The figure shows three views and two pictorial views of one solid part (mm, origin at its lowest corner). Answer the questions. A direction names the side the tool comes from. Round coordinates to 2 decimals unless told otherwise and drop trailing zeros. Answer as a JSON object with one key per item and string values. Group by question number.
Item 1: The mould has two halves that part along X. Classify the marked faces 4, 5 and 6: pulls with the +X half, pulls with the -X half, needs draft (parallel to the pull), parting line crosses it, or undercut.
Item 2: Section A-A, the plane z = 10 is taken. Count the separate pieces of the cut face and the enclosed holes in it, plus the area to 3 significant figures.
Item 3: Given P1, Ø11, axis at x = 7, y = 25.5, coming from the -Z side; P2, Ø6, axis at y = 24.5, z = 3.5, coming from the -X side; P3, Ø6, axis at x = 9.5, z = 6, coming from the -Y side, each flat-ended and moving along its own axis, determine where each tip first touches the part or whether it passes through.
Item 4: Consider probe 1 along Y at (x, z) = (28, 12.75); probe 2 along Z at (x, y) = (10, 13.5); probe 3 along Y at (x, z) = (5, 13.7). Determine where each line is inside the solid, lowest interval first. Write a range as from..to.
Item 5: For the marked faces 1, 2 and 3, determine the directions among +Z, -Z, +X, -X, +Y, -Y from which every point of the face is accessible in a straight line to the end or side of a thin tool.
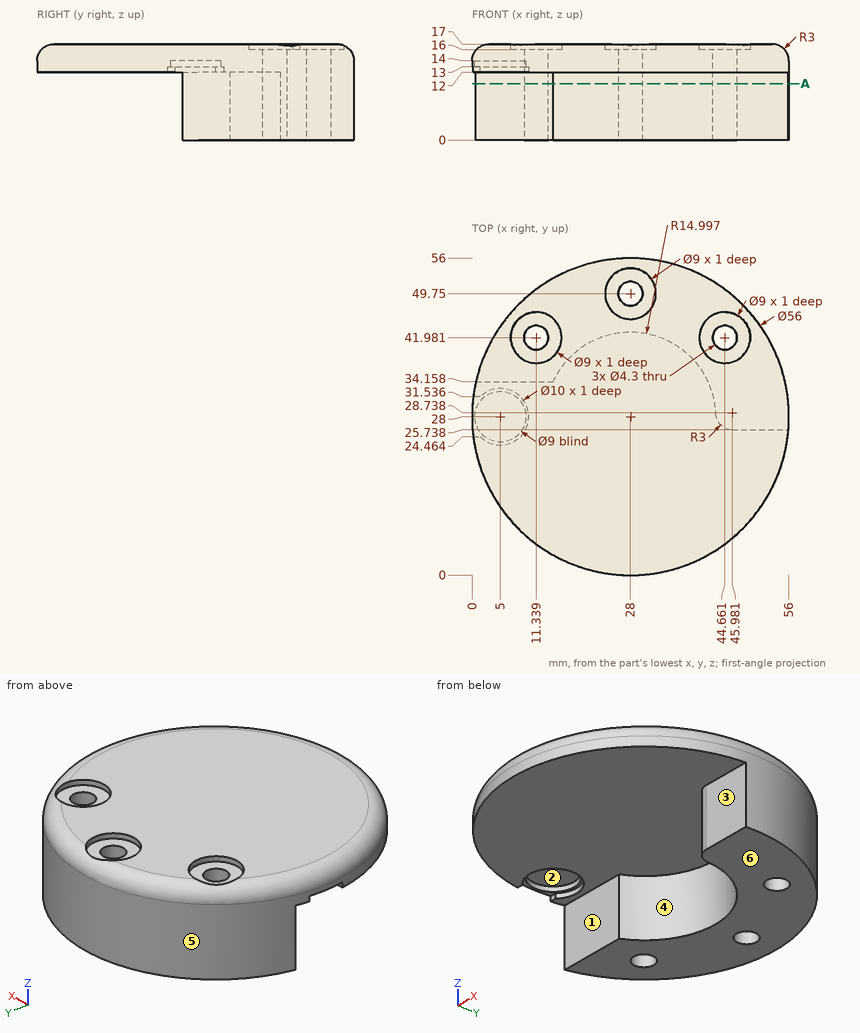
Values found:
{
 "1": {"face 4": "undercut", "face 5": "parting line crosses it", "face 6": "needs draft"},
 "2": {"separate pieces": "1", "enclosed holes": "3", "area": "781 mm2"},
 "3": {"P1": "z = 12", "P2": "x = 43.25", "P3": "y = 34.16"},
 "4": {"probe 1": "0..47.6, 51.9..56", "probe 2": "12..17", "probe 3": "12.03..23.5, 32.5..43.97"},
 "5": {"face 1": "-Z, -X, -Y", "face 2": "-Z", "face 3": "-Z, +X, -X, -Y"}
}
